Could you check a few things on this model? Use its own coordinates, in mm. A direction names the side the tool comes from. Give positions to 0.01 mm unless a question says otherwise; leave off trailing zeros. Order: outer loops, then holes, each group sorted by start corner. A loop starts at its lowest first (then second) coordinate and runs counter-clockwise, first axis right, second up. Notation, with made-up numbers: M 34,-24.5 L 61,-24.5 A33 ccw 61,13.5 Z; hole C -14,79.5 d2. An arc over 180 degrees is marked long. Use a Markdown table: item, result. Add a question column.
Autodesk Inventor part; units mm, degrees
ref_plane "YZ Plane" through (0, 0, 0) normal (1, 0, 0) x (0, 1, 0)
ref_plane "XZ Plane" through (0, 0, 0) normal (0, 1, 0) x (-1, 0, 0)
ref_plane "XY Plane" through (0, 0, 0) normal (0, 0, 1) x (1, 0, 0)
sketch "lock_sketch" plane through (0, 0, 0) normal (0, 0, 1) x (1, 0, 0)
  line L0 (0, 0) -> (10, 0)
  line L1 (10, 0) -> (10, 2.6)
  line L2 (0, 2.6) -> (10, 2.6)
  line L3 (0, 0) -> (0, 2.6)
  line L4 (0.2, -4) -> (9.8, -4) construction
  line L5 (9.8, -4) -> (9.8, 5.6) construction
  line L6 (9.8, 5.6) -> (0.2, 5.6)
  line L7 (0.2, 5.6) -> (0.2, -4) construction
  arc A0 (0.2, 5.6) -> (0.2, 2.6) centre (3.2, 4.1) ccw
  arc A1 (9.8, 2.6) -> (9.8, 5.6) centre (6.8, 4.1) ccw
  line L8 (5, -4) -> (5, 0) construction
  line L9 (9.8, 2.6) -> (9.8, 0)
  line L10 (0.2, 2.6) -> (0.2, 0)
  line L11 (0.2, 0) -> (0.2, 0)
  line L12 (-0.8, -1) -> (-0.8, -1)
  line L13 (2.2, -4) -> (7.8, -4)
  line L14 (10.8, -1) -> (10.8, -1)
  line L15 (9.8, 0) -> (9.8, 0)
  arc A2 (-0.8, -1) -> (2.2, -4) centre (2.2, -1) ccw
  arc A3 (7.8, -4) -> (10.8, -1) centre (7.8, -1) ccw
  arc A4 (0.2, 0) -> (-0.8, -1) centre (0.2, -1) ccw
  arc A5 (10.8, -1) -> (9.8, 0) centre (9.8, -1) ccw
  line L16 (2.2, 5.6) -> (3.5, -2)
  line L17 (3.5, -2) -> (6.5, -2)
  line L18 (6.5, -2) -> (7.8, 5.6)
  point P0 (-0.8, 0)
  point P1 (10.8, 0)
  point P2 (0.2, 0)
  point P3 (9.8, 0)
  point P4 (5, -4)
  dimension "d4" = 0
  dimension "d0" = 10
  dimension "d1" = 9.6
  dimension "d2" = 0.2
  dimension "d6" = 3
  dimension "d7" = 3
  dimension "d9" = 2
  dimension "d10" = 2
  dimension "d14" = 4
  dimension "d17" = 3
  dimension "d18" = 1
  dimension "d19" = 1
  dimension "d22" = 3
  dimension "d23" = 1
  dimension "d24" = 3
  dimension "d25" = 2
extrude "lock" add sketch "lock_sketch" along normal blind 2 contours L10 L2 L16 L0 | L0 L16 L17 L18 A5 A3 L13 A2 A4 | A0 L6 L16 L2 | L18 L2 L9 L0 | L18 L6 A1 L2
fillet "teeth" radius 1 4 edges at (2.2, 5.6, 1) (7.8, 5.6, 1) (0.2, 5.6, 1) (9.8, 5.6, 1)
fillet "inside" radius 1.8 2 edges at (3.5, -2, 1) (6.5, -2, 1)
equation "\"d2\" = -0.5 * d1 + 0.5 * d0"
equation "\"d7\" = d17"
equation "\"d25\" = 0.5 * d14"
properties part number "fastener_lock" material "ABS Plastic"
1) We'd pull the mould along Y, two halves only. Please class faces 1 (the face through (-0.515, -0.301, 0.986)), 2 (the face through (2.009, 5.358, 1.014)), 3 (the face through (4.9, -2.3, 2)), 4 (the face through (-0.126, 3.667, 0.986)): pulls with the +Y half, pulls with the -Y half, needs draft (parallel to the pull), parting line crosses it, or undercut.
2) For faces 5 (the face through (10.499, -0.285, 0.986)), 6 (the face through (0.2, 1, 1)), 7 (the face through (0.1, -3.14, 0.99)), 8 (the face through (7.2, 2.1, 1)), which set-ups out of +Z, -Z, +X, -X, +Y, -Y let a thin tool reach every point of the face, with its end or its side?
3) Suppose I cut it at A-A on y = 2.75. Please give me the cut outline in (x, z), and give its area (3 significant figures).
4) Please list where these lines run through material, in increasing order: line 1 (X direction, y = 3.25, z = 0.6); line 2 (X direction, y = 1, z = 0.25); line 3 (Y direction, x = 0.5, z = 1.75). Write a range as from..to.
5) Suppose I cut it at B-B on y = -0.25. Please give me the cut outline in (x, z), and give its area (3 significant figures).
6) For pin 1 (0.6 mm diameter, centred on y = 1.5, z = 1.5, fed in from -X); pin 2 (1 mm diameter, centred on y = 1.5, z = 0.5, fed in from +X), each with a flat end and sliding along its axis, tell me the tip position at first contact or that it passes through.
Values found:
| question | item | result |
|---|---|---|
| 1 | face 1 | undercut |
| 1 | face 2 | pulls with the +Y half |
| 1 | face 3 | needs draft |
| 1 | face 4 | undercut |
| 2 | face 5 | +Z, -Z, +X |
| 2 | face 6 | +Z, -Z, -X |
| 2 | face 7 | +Z, -Z, -X, -Y |
| 2 | face 8 | +Z, -Z, +Y |
| 3 | outline | M 0.13,0 L 2.69,0 L 2.69,2 L 0.13,2 Z; M 7.31,0 L 9.87,0 L 9.87,2 L 7.31,2 Z |
| 3 | area | 10.2 mm^2 |
| 4 | line 1 | x = -0.04..2.6, 7.4..10.04 |
| 4 | line 2 | x = 0.2..2.99, 7.01..9.8 |
| 4 | line 3 | y = -3.47..5.52 |
| 5 | outline | M -0.46,0 L 3.2,0 L 3.2,2 L -0.46,2 Z; M 6.8,0 L 10.46,0 L 10.46,2 L 6.8,2 Z |
| 5 | area | 14.6 mm^2 |
| 6 | pin 1 | stops at x = 0.2 |
| 6 | pin 2 | stops at x = 9.8 |
